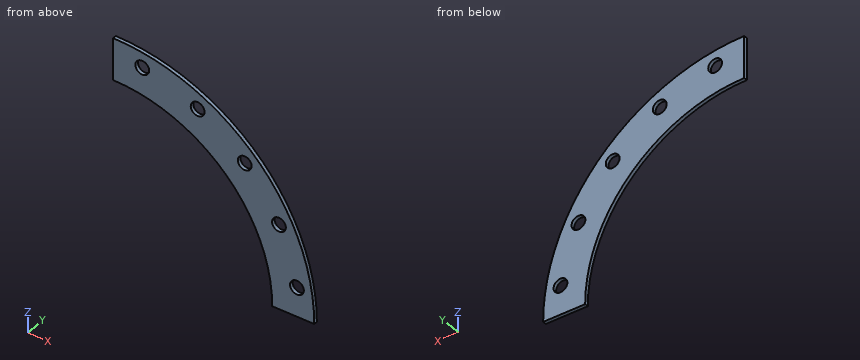
Autodesk Inventor part; units mm, degrees
ref_plane "YZ Plane" through (0, 0, 0) normal (1, 0, 0) x (0, 1, 0)
ref_plane "XZ Plane" through (0, 0, 0) normal (0, 1, 0) x (-1, 0, 0)
ref_plane "XY Plane" through (0, 0, 0) normal (0, 0, 1) x (1, 0, 0)
sketch "Sketch1" plane through (0, 0, 0) normal (0, 1, 0) x (-1, 0, 0)
  circle A0 centre (0, 0) radius 265
  circle A1 centre (0, 0) radius 335
  line L0 (335, 0) -> (265, 0)
  line L1 (-265, 0) -> (-335, 0)
  line L2 (0, 265) -> (0, 335)
  point P0 (300, 0)
  point P1 (-300, 0)
  point P2 (0, 300)
  dimension "d1" = 670
  dimension "d4" = 530
extrude "Extrusion1" add sketch "Sketch1" along normal blind 6 contours A0 L1 A1 L2
sketch "Sketch2" plane through (0, 0, 0) normal (0, -1, 0) x (1, 0, 0)
  arc A0 (335, 0) -> (0, 335) centre (0, 0) ccw
  line L0 (0, 265) -> (0, 335)
  arc A1 (265, 0) -> (0, 265) centre (0, 0) ccw
  line L1 (335, 0) -> (265, 0)
  circle A2 centre (48.4947, 306.1834) radius 11.5
  arc A3 (265, 0) -> (0, 265) centre (0, 0) ccw
  line L2 (48.4947, 306.1834) -> (0, 0)
  dimension "d5" = 310
  dimension "d6" = 9
  dimension "d7" = 23
extrude "Cut1" cut sketch "Sketch2" against normal blind 6 contours A2
pattern_circular "Circular Pattern1" count 20 over 360 about axis through (0, 0, 0) along (0, 1, 0) of "Cut1"
equation "\"d4\" = Accsess_hatch_diameter"
equation "\"d9\" = Thickness"
equation "\"BendRadius\" = Thickness"
equation "\"BendReliefWidth\" = Thickness"
equation "\"BendReliefDepth\" = 0.5 * Thickness"
equation "\"CornerReliefSize\" = 4 * Thickness"
equation "\"MinimumRemnant\" = 2 * Thickness"
equation "\"TransitionRadius\" = BendRadius"
equation "\"JacobiRadiusSize\" = BendRadius"
equation "\"GapSize\" = Thickness"
equation "\"d8\" = Thickness"
properties part number "PNS-712 accses hatch flangeipt" material "Steel"
For this review, take the finished solid that the model builds, in its own axes (mm). Coordinates: 2 decimals unless noted, no trailing zeros. Write each loop counter-clockwise with the first axis right and the second up, starting at its lowest first coordinate (ties: lowest second). Pieces come first, ordered by that corner, then holes. Notation, with made-up numbers: (37.25, -2) -> (41.25, -2) arc R13 ccw to (41.25, 15) -> close; hole circle Ø8 at (38, 57.5). An arc over 180 degrees is marked (long way). Put each result on its own line as item: value.
Q1. Wall thickness on L1, parallel to Z at x = 285, y = 3.85; L2, parallel to X at y = 2.3, z = 225; L3, parallel to Z at x = 57.5, y = 4.2: over which ranges is each line inside the solid? List them lowest first.
From the geometry:
L1: z = 0 to 133.32, 148.15 to 176.07
L2: x = 140 to 209.27, 229.14 to 248.19
L3: z = 258.69 to 299.03, 313.34 to 330.03
Q2. Take a section at A-A, the plane z = 53. State the section outline as (x, y) points, then the cut area to 3 significant figures.
From the geometry:
outline: (259.65, 0) -> (295.6, 0) -> (295.6, 6) -> (259.65, 6) -> close; (316.76, 0) -> (330.78, 0) -> (330.78, 6) -> (316.76, 6) -> close
area: 300 mm2
Q3. Take a section at D-D, the plane x = 200.5. State the section outline as (y, z) points.
From the geometry:
outline: (0, 173.28) -> (6, 173.28) -> (6, 268.37) -> (0, 268.37) -> close
Q4. Take a section at C-C, the plane x = 80.5. State the section outline as (y, z) points, then the cut area to 3 significant figures.
From the geometry:
outline: (0, 252.48) -> (6, 252.48) -> (6, 325.18) -> (0, 325.18) -> close
area: 436 mm2
Q5. Take a section at B-B, the plane y = 2.4. State the section outline as (x, z) points.
From the geometry:
outline: (0, 265) arc R265 cw to (265, 0) -> (335, 0) arc R335 ccw to (0, 335) -> close; hole circle Ø23 at (48.49, 306.18); hole circle Ø23 at (140.74, 276.21); hole circle Ø23 at (219.2, 219.2); hole circle Ø23 at (276.21, 140.74); hole circle Ø23 at (306.18, 48.49)
Q6. Clearance check with flat-ended pins moving along their axes: pin 1 Ø1.5 at (x, y) = (144.5, 2) entering from +Z; pin 2 Ø1 at (x, y) = (95, 4.5) entering from -Z; pin 3 Ø3 at (x, y) = (85.5, 1) entering from -Z. State where each tip first meets the part, or that it passes through.
From the geometry:
pin 1: stops at z = 302.59
pin 2: stops at z = 247.19
pin 3: stops at z = 250.31
